Autodesk Inventor part; units mm, degrees
ref_plane "YZ Plane" through (0, 0, 0) normal (1, 0, 0) x (0, 1, 0)
ref_plane "XZ Plane" through (0, 0, 0) normal (0, 1, 0) x (-1, 0, 0)
ref_plane "XY Plane" through (0, 0, 0) normal (0, 0, 1) x (1, 0, 0)
sketch "Sketch1" plane through (0, 0, 0) normal (0, 0, 1) x (1, 0, 0)
  line L0 (-11.7555, 11.7555) -> (11.7555, 11.7555)
  line L1 (11.7555, 11.7555) -> (11.7555, -8.812)
  line L2 (8.812, -11.7555) -> (-8.812, -11.7555)
  line L3 (-11.7555, -8.812) -> (-11.7555, 11.7555)
  line L4 (-11.7555, 11.7555) -> (11.7555, -11.7555) construction
  line L5 (11.7555, 11.7555) -> (-11.7555, -11.7555) construction
  line L6 (11.7555, -11.7555) -> (8.812, -11.7555)
  line L7 (8.812, -11.7555) -> (8.812, -8.812)
  line L8 (8.812, -8.812) -> (11.7555, -8.812)
  line L9 (11.7555, -8.812) -> (11.7555, -11.7555)
  line L10 (-8.812, -11.7555) -> (-8.812, -8.812)
  line L11 (-8.812, -8.812) -> (-11.7555, -8.812)
  circle A0 centre (0, 0) radius 6.35
  point P0 (0, 0)
  dimension "d4" = 12.7
extrude "Extrusion1" add sketch "Sketch1" along normal blind 25.4 contours L0 L1 L8 L7 L2 L10 L11 L3
mirror "Mirror1" about plane through (0, 0, 0) normal (1, 0, 0)
sketch "Sketch3" plane through (-11.7555, -8.812, 0) normal (-1, 0, 0) x (0, 0, 1)
  circle A0 centre (12.3172, 9.3487) radius 5.08
  point P0 (0, 8.812)
  dimension "d13" = 10.16
extrude "Extrusion3" add sketch "Sketch3" along normal blind 10.16
sketch "Sketch4" plane through (-11.7555, 11.7555, 0) normal (0, 1, 0) x (1, 0, 0)
  line L0 (23.5109, 0) -> (23.5109, -25.4)
  line L1 (0, 0) -> (2.9435, 0)
  line L2 (23.5109, -25.4) -> (0, -25.4)
  line L3 (0, -25.4) -> (0, 0)
  line L4 (0, 0) -> (23.5109, 0)
  line L5 (23.5109, 0) -> (23.5109, -25.4)
  point P0 (11.7555, 0)
  point P1 (2.9435, 0)
extrude "Extrusion4" add sketch "Sketch4" along normal blind 50.8
sketch "Sketch5" plane through (11.7555, -8.812, 25.4) normal (1, 0, 0) x (0, 0, -1)
  line L0 (25.4, 0) -> (0, 0)
  line L1 (25.4, 0) -> (25.4, 71.3674)
  line L2 (0, 0) -> (25.4, 0)
  line L3 (25.4, 0) -> (25.4, 71.3674)
  line L4 (25.4, 71.3674) -> (0, 71.3674)
  line L5 (0, 71.3674) -> (0, 0)
  point P0 (25.4, 8.812)
extrude "Extrusion5" add sketch "Sketch5" along normal blind 25.4
ref_plane "Work Plane1" through (0, 0, 0) normal (1, 0, 0) x (0, 1, 0)
equation "\"BendRadius\" = Thickness"
equation "\"BendReliefWidth\" = Thickness"
equation "\"BendReliefDepth\" = 0.5 * Thickness"
equation "\"CornerReliefSize\" = 4 * Thickness"
equation "\"MinimumRemnant\" = 2 * Thickness"
equation "\"TransitionRadius\" = BendRadius"
equation "\"JacobiRadiusSize\" = BendRadius"
equation "\"GapSize\" = Thickness"
properties part number "new slider part"
Could you check a few things on this model? Use its own coordinates, in mm. A direction names the side the tool comes from. Give positions to 0.01 mm unless a question says otherwise; leave off trailing zeros. Order: outer loops, then holes, each group sorted by start corner. A loop starts at its lowest first (then second) coordinate and runs counter-clockwise, first axis right, second up.
1. Suppose I cut it at B-B (z = 13.5). Write out the boundary of the cut face in (x, y).
Answers below:
outline: (-21.92, -4.4) - (-11.76, -4.4) - (-11.76, -8.81) - (-8.81, -8.81) - (-8.81, -11.76) - (8.81, -11.76) - (8.81, -8.81) - (37.16, -8.81) - (37.16, 62.56) - (-11.76, 62.56) - (-11.76, 5.48) - (-21.92, 5.48) - close; hole circle Ø12.7 at (0, 0)
2. Suppose I cut it at C-C (y = 54). Write out the boundary of the cut face in (x, z).
Answers below:
outline: (-11.76, 0) - (37.16, 0) - (37.16, 25.4) - (-11.76, 25.4) - close
3. Thinking about a two-plate mould opening in Y: for faces 4 (the cylindrical face through (-1.38, 6.2, 12.52)), 5 (the flat face through (0, -11.756, 13)), 6 (the flat face through (12, 25, 0)), 7 (the cylindrical face through (-16.76, 3.63, 8.29)), which applies, +Y half, -Y half, draft (parallel to the pull), parting line (faces both ways), or undercut?
Answers below:
face 4: undercut
face 5: -Y half
face 6: draft
face 7: parting line
4. For pin 1 (1 mm diameter, centred on y = 31, z = 7, fed in from -X); pin 2 (2 mm diameter, centred on x = -14.5, z = 22.5, fed in from -Y); pin 3 (0.9 mm diameter, centred on y = -10.5, z = 6.5, fed in from -X); pin 4 (0.9 mm diameter, centred on x = -10, z = 13.5, fed in from -Y), each with a flat end and sliding along its axis, tell me the tip position at first contact or that it passes through.
Answers below:
pin 1: stops at x = -11.76
pin 2: passes through
pin 3: stops at x = -8.81
pin 4: stops at y = -8.81
5. Suppose I cut it at A-A (x = 0). Write out the boundary of the cut face in (y, z).
Answers below:
outline: (-11.76, 0) - (-6.35, 0) - (-6.35, 25.4) - (-11.76, 25.4) - close; (6.35, 0) - (62.56, 0) - (62.56, 25.4) - (6.35, 25.4) - close
6. I need wall thicknesses on L1, parallel to X at y = 0, z = 19.5; L2, parallel to X at y = 0, z = 8.5; L3, parallel to Y at x = 0, z = 8. Which ranges of each line are inside material? Lowest first, please.
Answers below:
L1: x = -11.76 to -6.35, 6.35 to 37.16
L2: x = -21.92 to -6.35, 6.35 to 37.16
L3: y = -11.76 to -6.35, 6.35 to 62.56
7. Which directions (+Z, -Z, +X, -X, +Y, -Y) give clear straight access to the entire face, cutting with the end or side of a thin tool? Please do faces 1 (the flat face through (-10, -8.812, 13)), 2 (the flat face through (37.156, 27, 13)), 3 (the flat face through (8.812, -10, 13)).
Answers below:
face 1: +Z, -Z, -X, -Y
face 2: +Z, -Z, +X, +Y, -Y
face 3: +Z, -Z, +X, -Y
8. Suppose I cut it at D-D (x = 29). Write out the boundary of the cut face in (y, z).
Answers below:
outline: (-8.81, 0) - (62.56, 0) - (62.56, 25.4) - (-8.81, 25.4) - close
